```python
from build123d import *

# Parameters (mm, degrees)
CYLINDER040_R          = 4.2
CYLINDER040_DEPTH      = 200
CYLINDER037_R          = 1.8
CYLINDER037_DEPTH      = 21
CYLINDER037_ROLL_ANGLE = 90
BOX009_W               = 19
BOX009_H               = 14
BOX009_DEPTH           = 10
BOX008_W               = 45
BOX008_H               = 20
BOX008_DEPTH           = 10


with BuildPart() as cilindro037:
    # Cylinder040 → Cylinder040 (new body)
    with BuildSketch(Plane(origin=(57, -40, -29), x_dir=(1, 0, 0), z_dir=(0, 0, 1))):
        Circle(CYLINDER040_R)
    extrude(amount=CYLINDER040_DEPTH)


with BuildPart() as cilindro034:
    # Cylinder037 → Cylinder037 (new body)
    with BuildSketch(Plane.XY):
        Circle(CYLINDER037_R)
    extrude(amount=CYLINDER037_DEPTH)


with BuildPart() as cilindro034_1:
    # Cylinder037 roll: moved
    add(cilindro034.part.rotate(Axis((0, 0, 0), (1, 0, 0)), CYLINDER037_ROLL_ANGLE))


with BuildPart() as cilindro034_2:
    # Cylinder037 placement: moved
    add(cilindro034_1.part.moved(Location((88, -32, 22))))


with BuildPart() as cubo009:
    # Box009 → Box009 (new body)
    with BuildSketch(Plane(origin=(74, -43, 17), x_dir=(1, 0, 0), z_dir=(0, 0, 1))):
        with Locations((9.5, 7)):
            Rectangle(BOX009_W, BOX009_H)
    extrude(amount=BOX009_DEPTH)


with BuildPart() as parte_superior:
    # Box008 → Box008 (new body)
    with BuildSketch(Plane(origin=(48, -50, 17), x_dir=(1, 0, 0), z_dir=(0, 0, 1))):
        with Locations((22.5, 10)):
            Rectangle(BOX008_W, BOX008_H)
    extrude(amount=BOX008_DEPTH)

    # Cut037: cut Cubo009
    add(cubo009.part, mode=Mode.SUBTRACT)

    # Cut038: cut Cilindro034
    add(cilindro034_2.part, mode=Mode.SUBTRACT)


with BuildPart() as parte_superior_1:
    # Cut038 placement: moved
    add(parte_superior.part.moved(Location((0, 0, 146))))

    # Cut039: cut Cilindro037
    add(cilindro037.part, mode=Mode.SUBTRACT)


solid = parte_superior_1.part
```
CAD build for the part. Positions are in the model's coordinates, mm. A direction names the side the tool comes from. Give positions to 0.01 mm unless a question says otherwise; leave off trailing zeros. Write each loop counter-clockwise with the first axis right and the second up, starting at its lowest first coordinate (ties: lowest second). Pieces come first, ordered by that corner, then holes. Notation, with made-up numbers: M -29.75,-34 L -18.75,-34 A17 cw -18.75,-30 Z; hole C 63,-23 d10. An arc over 180 degrees is marked long. Return JSON: item names as keys, results as strings. Group by question number.
(1) Mould opens along Y. For faces 3 (the face through (53.904, -37.161, 166.944)), 4 (the face through (83, -43, 168)), 5 (the face through (70, -50, 168)), 6 (the face through (74, -37, 168)) say: pulls with the +Y half, pulls with the -Y half, needs draft (parallel to the pull), parting line crosses it, or undercut.
(2) Band-saw the part on B-B (x = 88). Give the cut face in (y, z).
(3) Drill centre lines: L1, parallel to X at y = -45, z = 168; L2, parallel to Z at x = 88, y = -47; L3, parallel to X at y = -40, z = 166. Where is each one in solid material? Low to high. Write a range as [from, to].
(4) Flat gauge pins, fed straight in: pin 1 Ø3 at (y, z) = (-37.5, 169.5) entering from +X; pin 2 Ø2 at (x, z) = (88, 168) entering from -Y; pin 3 Ø5 at (x, z) = (83.5, 169) entering from +Y; pin 4 Ø2.5 at (x, y) = (58.5, -41.5) entering from -Z. Where does each tip first touch, or does it go through?
(5) 3-axis set-ups, long thin cutter, end or side, ignore diameter. For faces 1 (the face through (48, -40, 168)), 2 (the face through (57, -40, 171)): which of +Z, -Z, +X, -X, +Y, -Y reach the whole face in a straight line?
(6) Band-saw the part on C-C (y = -40). Give the cut face in (x, z), and give its area (3 significant figures).
(7) Band-saw the part on A-A (z = 168). Give the cut face in (x, y).
(8) Band-saw the part on D-D (y = -45.75). Give the cut face in (x, z).
Entries:
{
 "1": {"face 3": "undercut", "face 4": "pulls with the +Y half", "face 5": "pulls with the -Y half", "face 6": "needs draft"},
 "2": {"outline": "M -50,163 L -43,163 L -43,166.2 L -50,166.2 Z; M -50,169.8 L -43,169.8 L -43,173 L -50,173 Z"},
 "3": {"L1": "x = [48, 86.2], [89.8, 93]", "L2": "z = [163, 166.2], [169.8, 173]", "L3": "x = [48, 52.8], [61.2, 74]"},
 "4": {"pin 1": "stops at x = 74", "pin 2": "passes through", "pin 3": "stops at y = -43", "pin 4": "stops at z = 171"},
 "5": {"face 1": "+Z, -Z, -X, +Y, -Y", "face 2": "-Z"},
 "6": {"outline": "M 48,163 L 52.8,163 L 52.8,171 L 61.2,171 L 61.2,163 L 74,163 L 74,173 L 48,173 Z", "area": "193 mm^2"},
 "7": {"outline": "M 48,-50 L 86.2,-50 L 86.2,-43 L 74,-43 L 74,-30 L 48,-30 Z; M 89.8,-50 L 93,-50 L 93,-43 L 89.8,-43 Z; hole C 57,-40 d8.4"},
 "8": {"outline": "M 48,163 L 93,163 L 93,173 L 48,173 Z; hole C 88,168 d3.6"}
}
